from build123d import *

# Parameters (mm, degrees)
F0_W     = 35.56
F0_H     = 35.56
F1_DEPTH = 5.08
F2_W     = 19.812
F2_H     = 4.572
F3_DEPTH = 2.54
F4_W     = 20.32
F4_H     = 5.08
F5_DEPTH = 2.54
F6_W     = 20.32
F6_H     = 5.08
F7_DEPTH = 2.54
F8_W     = 20.32
F8_H     = 5.08
F9_DEPTH = 2.54


with BuildPart() as f1:
    # F0 (on Top) → F1 (new body, symmetric)
    with BuildSketch(Plane.XY):
        Rectangle(F0_W, F0_H)
        with BuildLine():
            Line((-8.8966145833, -12.7), (-8.8966145833, 12.4850260417))
            Line((-8.8966145833, 12.4850260417), (-1.0583333333, 12.4850260417))
            add(Edge.make_bspline(
                [(-1.0583333333, 12.4850260417), (4.2994791667, 12.4850260417), (6.7193142361, 10.9609157986)],
                knots=[0, 0, 0, 1, 1, 1], degree=2))
            add(Edge.make_bspline(
                [(6.7193142361, 10.9609157986), (9.1391493056, 9.4368055556), (9.1391493056, 6.1129774306)],
                knots=[0, 0, 0, 1, 1, 1], degree=2))
            add(Edge.make_bspline(
                [(9.1391493056, 6.1129774306), (9.1391493056, 3.8529947917), (8.0808159722, 2.4060546875)],
                knots=[0, 0, 0, 1, 1, 1], degree=2))
            add(Edge.make_bspline(
                [(8.0808159722, 2.4060546875), (7.0224826389, 0.9591145833), (5.2641059028, 0.6669704861)],
                knots=[0, 0, 0, 1, 1, 1], degree=2))
            Line((5.2641059028, 0.6669704861), (5.2641059028, 0.49609375))
            add(Edge.make_bspline(
                [(5.2641059028, 0.49609375), (7.6563802083, -0.0385850694), (8.7174696181, -1.5020616319)],
                knots=[0, 0, 0, 1, 1, 1], degree=2))
            add(Edge.make_bspline(
                [(8.7174696181, -1.5020616319), (9.7785590278, -2.9655381944), (9.7785590278, -5.3963975694)],
                knots=[0, 0, 0, 1, 1, 1], degree=2))
            add(Edge.make_bspline(
                [(9.7785590278, -5.3963975694), (9.7785590278, -8.8414930556), (7.2870659722, -10.7707465278)],
                knots=[0, 0, 0, 1, 1, 1], degree=2))
            add(Edge.make_bspline(
                [(7.2870659722, -10.7707465278), (4.7955729167, -12.7), (0.5236545139, -12.7)],
                knots=[0, 0, 0, 1, 1, 1], degree=2))
            Line((0.5236545139, -12.7), (-8.8966145833, -12.7))
        make_face(mode=Mode.SUBTRACT)
    extrude(amount=F1_DEPTH, both=True)

    # F2 (on face) → F3 (join)
    with BuildSketch(Plane(origin=(0, 17.78, 0), x_dir=(-1, 0, 0), z_dir=(0, 1, 0))):
        Rectangle(F2_W, F2_H)
    extrude(amount=F3_DEPTH)

    # F4 (on face) → F5 (join)
    with BuildSketch(Plane(origin=(-17.78, 0, 0), x_dir=(0, -1, 0), z_dir=(-1, 0, 0))):
        Rectangle(F4_W, F4_H)
    extrude(amount=F5_DEPTH)

    # F6 (on face) → F7 (cut)
    with BuildSketch(Plane.XZ.offset(17.78)):
        Rectangle(F6_W, F6_H)
    extrude(amount=-F7_DEPTH, mode=Mode.SUBTRACT)

    # F8 (on face) → F9 (cut)
    with BuildSketch(Plane.YZ.offset(17.78)):
        Rectangle(F8_W, F8_H)
    extrude(amount=-F9_DEPTH, mode=Mode.SUBTRACT)


solid = f1.part
Check sheet for the modelled part. Datum: model origin and axes. Units: mm. A direction names the side the tool comes from. Give positions to 0.01 mm unless a question says otherwise; leave off trailing zeros. Write each loop counter-clockwise with the first axis right and the second up, starting at its lowest first coordinate (ties: lowest second). Pieces come first, ordered by that corner, then holes. Notation, with made-up numbers: (73, -39) -> (128, -39) arc R27 cw to (128, 0) -> close; hole circle Ø2 at (59, 51). An arc over 180 degrees is marked (long way). One line per item, written item: value. Start each with the question number.
Item 1: Material ranges on probe 1 along Y at (x, z) = (-4.5, -3.25); probe 2 along Y at (x, z) = (-1, -0.5); probe 3 along X at (y, z) = (-14.5, -1.75), recorded low to high. Write a range as from..to.
Item 2: Section check A-A on y = 15. Record the cut outline in (x, z).
Item 3: Tool access check on faces 1 (the flat face through (17, -10.16, 0)), 2 (the flat face through (-8.897, 0, 0)), 3 (the flat face through (-19, -10.16, 0)). Record the directions out of +Z, -Z, +X, -X, +Y, -Y that give a thin tool (end or side, any length) a straight path to the whole face; none if there is none.
Item 4: Draft check along Z on faces 4 (the flat face through (0, 17.78, 3)), 5 (the flat face through (0, 19, 2.286)), 6 (the flat face through (0, -15.24, 0)), 7 (the flat face through (0, 19, -2.286)). Enter one of: +Z half, -Z half, draft (parallel to the pull), parting line (faces both ways), or undercut.
Item 5: Gauge pin test, flat ends, axial feed: pin 1 (1.3 mm diameter, centred on x = -19.5, z = 0.5, fed in from +Y); pin 2 (2 mm diameter, centred on x = 1.5, y = 19, fed in from +Z); pin 3 (2 mm diameter, centred on x = 16.5, z = -0.5, fed in from +Y). Record the tip position at first contact, or that the pin passes through.
Results list:
1. probe 1: -17.78..-12.7, 12.49..17.78
1. probe 2: -15.24..-12.7, 12.48..20.32
1. probe 3: -17.78..17.78
2. outline: (-17.78, -5.08) -> (17.78, -5.08) -> (17.78, 5.08) -> (-17.78, 5.08) -> close
3. face 1: +X
3. face 2: +Z, -Z
3. face 3: +Z, -Z, -X, -Y
4. face 4: draft
4. face 5: +Z half
4. face 6: undercut
4. face 7: -Z half
5. pin 1: y = 10.16
5. pin 2: z = 2.29
5. pin 3: y = 17.78
